```python
from build123d import *

# Parameters (mm, degrees)
SKETCH1_R           = 3.3655
SKETCH1_R_2         = 2.2352
BOSS_EXTRUDE1_DEPTH = 2.54
SKETCH2_R           = 0.6604
SKETCH2_R_2         = 2.31775
SKETCH2_R_3         = 3.3655
SKETCH2_R_4         = 2.2352
SKETCH2_R_5         = 1.143
BOSS_EXTRUDE2_DEPTH = 1.7272
FILLET1_R           = 12.7
SKETCH3_R           = 2.06375
SKETCH3_R_2         = 1.143
CUT_EXTRUDE1_DEPTH  = 1.27


with BuildPart() as part:
    # Sketch1 → Boss-Extrude1 (new body)
    with BuildSketch(Plane(origin=(0, 0, 0), x_dir=(1, 0, 0), z_dir=(0, 1, 0))):
        with Locations(Location((0, 0, 0), (0, 0, 270))):
            Circle(SKETCH1_R)
        with Locations(Location((0, 0, 0), (0, 0, 270))):
            Circle(SKETCH1_R_2, mode=Mode.SUBTRACT)
    extrude(amount=BOSS_EXTRUDE1_DEPTH)

    # Sketch2 → Boss-Extrude2 (add)
    with BuildSketch(Plane(origin=(0, 2.54, 0), x_dir=(1, 0, 0), z_dir=(0, 1, 0))):
        with BuildLine():
            ThreePointArc((-0.713521748, -3.755518873), (-3.8227, 0), (-0.713521748, 3.755518873))
            Line((-0.713521748, 3.755518873), (-16.092265178, 2.307544345))
            ThreePointArc((-16.092265178, 2.307544345), (-14.314807913, 1.713991165), (-13.55725, 0))
            ThreePointArc((-13.55725, 0), (-14.314807913, -1.713991165), (-16.092265178, -2.307544345))
            Line((-16.092265178, -2.307544345), (-0.713521748, -3.755518873))
        make_face()
        with Locations(Location((-12.8778, 0, 0), (0, 0, 270))):
            Circle(SKETCH2_R, mode=Mode.SUBTRACT)
        with Locations(Location((-9.8806, 0, 0), (0, 0, 270))):
            Circle(SKETCH2_R, mode=Mode.SUBTRACT)
        with Locations(Location((-7.1628, 0, 0), (0, 0, 270))):
            Circle(SKETCH2_R, mode=Mode.SUBTRACT)
        with Locations((-15.875, 0)):
            Circle(SKETCH2_R_2)
        with Locations(Location((-15.875, 0, 0), (0, 0, 270))):
            Circle(SKETCH2_R, mode=Mode.SUBTRACT)
        with BuildLine():
            Line((16.092265178, 2.307544345), (0.713521748, 3.755518873))
            ThreePointArc((0.713521748, 3.755518873), (2.944538578, 2.437771083), (3.8227, 0))
            ThreePointArc((3.8227, 0), (2.944538578, -2.437771083), (0.713521748, -3.755518873))
            Line((0.713521748, -3.755518873), (16.092265178, -2.307544345))
            ThreePointArc((16.092265178, -2.307544345), (13.55725, 0), (16.092265178, 2.307544345))
        make_face()
        with Locations(Location((7.1628, 0, 0), (0, 0, 270))):
            Circle(SKETCH2_R, mode=Mode.SUBTRACT)
        with Locations(Location((9.8806, 0, 0), (0, 0, 270))):
            Circle(SKETCH2_R, mode=Mode.SUBTRACT)
        with Locations(Location((12.8778, 0, 0), (0, 0, 270))):
            Circle(SKETCH2_R, mode=Mode.SUBTRACT)
        with Locations((15.875, 0)):
            Circle(SKETCH2_R_2)
        with Locations(Location((15.875, 0, 0), (0, 0, 270))):
            Circle(SKETCH2_R, mode=Mode.SUBTRACT)
        with BuildLine():
            Line((0.713521748, 3.755518873), (0, 3.8227))
            Line((0, 3.8227), (-0.713521748, 3.755518873))
            ThreePointArc((-0.713521748, 3.755518873), (-3.8227, 0), (-0.713521748, -3.755518873))
            Line((-0.713521748, -3.755518873), (0, -3.8227))
            Line((0, -3.8227), (0.713521748, -3.755518873))
            ThreePointArc((0.713521748, -3.755518873), (2.944538578, -2.437771083), (3.8227, 0))
            ThreePointArc((3.8227, 0), (2.944538578, 2.437771083), (0.713521748, 3.755518873))
        make_face()
        with Locations(Location((0, 0, 0), (0, 0, 270))):
            Circle(SKETCH2_R_3, mode=Mode.SUBTRACT)
        with Locations(Location((0, 0, 0), (0, 0, 270))):
            Circle(SKETCH2_R_3)
        with Locations(Location((0, 0, 0), (0, 0, 270))):
            Circle(SKETCH2_R_4, mode=Mode.SUBTRACT)
        with Locations(Location((0, 0, 0), (0, 0, 270))):
            Circle(SKETCH2_R_4)
        with Locations(Location((0, 0, 0), (0, 0, 270))):
            Circle(SKETCH2_R_5, mode=Mode.SUBTRACT)
    extrude(amount=BOSS_EXTRUDE2_DEPTH)

    # Fillet1
    fillet1_edges = [part.edges().sort_by_distance(p)[0] for p in [
        (0, 3.4036, -3.8227),
        (0, 3.4036, 3.8227),
    ]]
    fillet(fillet1_edges, radius=FILLET1_R)

    # Sketch3 → Cut-Extrude1 (cut)
    with BuildSketch(Plane(origin=(0, 4.2672, 0), x_dir=(1, 0, 0), z_dir=(0, 1, 0))):
        with Locations(Location((0, 0, 0), (0, 0, 270))):
            Circle(SKETCH3_R)
        with Locations(Location((0, 0, 0), (0, 0, 270))):
            Circle(SKETCH3_R_2, mode=Mode.SUBTRACT)
    extrude(amount=-CUT_EXTRUDE1_DEPTH, mode=Mode.SUBTRACT)


solid = part.part
```
The listing builds one solid part. Answer for the finished solid, in the listing's coordinates (mm). A direction names the side the tool comes from. Give positions to 0.01 mm unless a question says otherwise; leave off trailing zeros. Order: outer loops, then holes, each group sorted by start corner. A loop starts at its lowest first (then second) coordinate and runs counter-clockwise, first axis right, second up. Notation, with made-up numbers: (-30.75, 47) -> (26.25, 47) arc R19 cw to (26.25, 54) -> close; hole circle Ø4 at (30.25, 38). An arc over 180 degrees is marked (long way). Write each question's results on one line, items separated by ' | '.
Q1. Each of these flat-tipped pins is pushed along its axis until it touches: P1, Ø3.5, axis at x = 0, z = 0, coming from the +Y side; P2, Ø2, axis at x = -0.5, y = 1, coming from the -Z side. Where does it stop, or does it pass through?
Checked values:
P1: stops at y = 3 | P2: stops at z = -3.37
Q2. Determine the mould class of faces 4 (the face through (8.75, 3.39, -3)), 5 (the face through (-8.75, 3.39, 3)), 6 (the face through (13.32, 3.39, -0.49)) for opening direction X: pulls with the +X half, pulls with the -X half, needs draft (parallel to the pull), parting line crosses it, or undercut.
Checked values:
face 4: pulls with the +X half | face 5: pulls with the -X half | face 6: undercut
Q3. The part is cut by section D-D, the plane x = -11.5. Give the vertices of the cut face in (y, z), and give its area (3 significant figures).
Checked values:
outline: (2.54, -2.74) -> (4.27, -2.74) -> (4.27, 2.74) -> (2.54, 2.74) -> close | area: 9.46 mm^2
Q4. Straight lines are drawn through the part: probe 1 along X at (y, z) = (0.9, 0); probe 2 along Y at (x, z) = (-15, 0.5); probe 3 along X at (y, z) = (2.4, 1). For each, find the intervals that lie inside material, in ascending order. Write a range as from..to.
Checked values:
probe 1: x = -3.37..-2.24, 2.24..3.37 | probe 2: y = 2.54..4.27 | probe 3: x = -3.21..-2, 2..3.21
Q5. The part is cut by section A-A, the plane y = 1.9. Give the vertices of the cut face in (x, z).
Checked values:
outline: circle Ø6.73 at (0, 0); hole circle Ø4.47 at (0, 0)
Q6. Which of the six approach directions +Z, -Z, +X, -X, +Y, -Y give full straight-line access (tool end or side, diameter ignored) to faces 1 (the face through (2.838, 1.252, 1.809)), 2 (the face through (-18.192, 3.392, -0.048)), 3 (the face through (-1, 2.997, 1))?
Checked values:
face 1: -Y | face 2: -X, +Y, -Y | face 3: +Y
Q7. The part is cut by section B-B, the plane z = 0. State how many separate pieces and enclosed holes the cut face has, and give its area (3 significant figures).
Checked values:
separate pieces: 10 | enclosed holes: 0 | area: 44.0 mm^2
